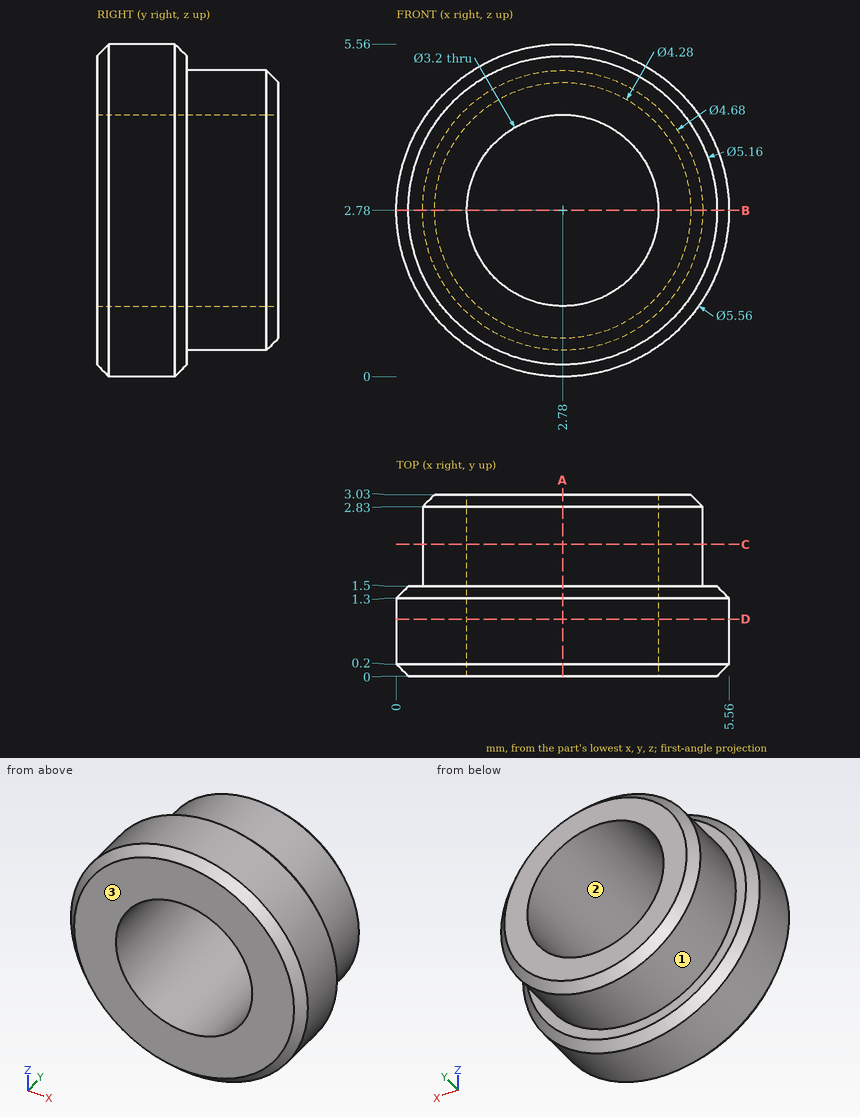
Geometry: see drawing. Coordinates: mm, zero at the bounding-box minimum. Give positions to 0.01 mm unless a question says otherwise; leave off trailing zeros. Write each loop counter-clockwise with the first axis right and the second up, starting at its lowest first coordinate (ties: lowest second). Pieces come first, ordered by that corner, then holes. Notation, with made-up numbers: M -40,52 L -29,52 A23 ccw -29,86 Z; hole C -10.75,-7.5 d7. An arc over 180 degrees is marked long. Return JSON: item names as keys, results as strings. Group by question number.
1) Ray query, L1, parallel to X at y = 1.6, z = 2.78; L2, parallel to X at y = 0.6, z = 2.78. Return the intervals inside material, ascending.
2) Cut plane C-C, the plane y = 2.2. Output: boundary loops of the cut face in (x, z), then the cut area to 3 significant figures.
3) Cut plane B-B, the plane z = 2.78. Output: boundary loops of the cut face in (x, y).
4) Draft query along X for the marked faces 1, 2 and 3. Return one class per face: released by +X, released by -X, zero draft, split by the parting line, or undercut.
5) Cut plane A-A, the plane x = 2.78. Output: boundary loops of the cut face in (y, z), then the cut area to 3 significant figures.
6) First-contact query: pin 1 Ø2.5 at (x, z) = (2.78, 2.78) entering from +Y. Flat tip, straight axial feed; report the tip coordinate or a pass-through.
7) Cut plane D-D, the plane y = 0.95. Output: boundary loops of the cut face in (x, z).
Data:
{
 "1": {"L1": "x = 0.44 to 1.18, 4.38 to 5.12", "L2": "x = 0 to 1.18, 4.38 to 5.56"},
 "2": {"outline": "C 2.78,2.78 d4.68; hole C 2.78,2.78 d3.2", "area": "9.16 mm²"},
 "3": {"outline": "M 0,0.2 L 0.2,0 L 1.18,0 L 1.18,3.03 L 0.64,3.03 L 0.44,2.83 L 0.44,1.5 L 0.2,1.5 L 0,1.3 Z; M 4.38,0 L 5.36,0 L 5.56,0.2 L 5.56,1.3 L 5.36,1.5 L 5.12,1.5 L 5.12,2.83 L 4.92,3.03 L 4.38,3.03 Z"},
 "4": {"face 1": "split by the parting line", "face 2": "undercut", "face 3": "zero draft"},
 "5": {"outline": "M 0,0.2 L 0.2,0 L 1.3,0 L 1.5,0.2 L 1.5,0.44 L 2.83,0.44 L 3.03,0.64 L 3.03,1.18 L 0,1.18 Z; M 0,4.38 L 3.03,4.38 L 3.03,4.92 L 2.83,5.12 L 1.5,5.12 L 1.5,5.36 L 1.3,5.56 L 0.2,5.56 L 0,5.36 Z", "area": "5.68 mm²"},
 "6": {"pin 1": "passes through"},
 "7": {"outline": "C 2.78,2.78 d5.56; hole C 2.78,2.78 d3.2"}
}
